from build123d import *

# Parameters (mm, degrees)
SKETCH1_R           = 45
BOSS_EXTRUDE1_DEPTH = 10
SKETCH3_R           = 2.1
CUT_EXTRUDE2_DEPTH  = 65.420493634
CIRPATTERN1_COUNT   = 4
SKETCH4_W           = 20
SKETCH4_H           = 20
CUT_EXTRUDE3_DEPTH  = 10
SKETCH6_R           = 2.55
CUT_EXTRUDE4_DEPTH  = 65.420493634


with BuildPart() as part:
    # Sketch1 → Boss-Extrude1 (new body)
    with BuildSketch(Plane(origin=(0, 0, 0), x_dir=(1, 0, 0), z_dir=(0, 1, 0))):
        with Locations(Location((0, 0, 0), (0, 0, 270))):
            Circle(SKETCH1_R)
    extrude(amount=BOSS_EXTRUDE1_DEPTH)

    # Sketch3 → Cut-Extrude2 (cut, through all)
    with BuildSketch(Plane(origin=(0, 10, 0), x_dir=(1, 0, 0), z_dir=(0, 1, 0))):
        with Locations(Location((0, 25, 0), (0, 0, 270))):
            Circle(SKETCH3_R)
    cut_extrude2 = extrude(amount=-CUT_EXTRUDE2_DEPTH, mode=Mode.SUBTRACT)

    # CirPattern1: Cut-Extrude2 ×4 about axis
    cirpattern1_axis = Axis((0, 0, 0), (0, 1, 0))
    for i in range(1, CIRPATTERN1_COUNT):
        add(cut_extrude2.rotate(cirpattern1_axis, i * 360 / CIRPATTERN1_COUNT), mode=Mode.SUBTRACT)

    # Sketch4 → Cut-Extrude3 (cut)
    with BuildSketch(Plane(origin=(0, 10, 0), x_dir=(1, 0, 0), z_dir=(0, 1, 0))):
        Rectangle(SKETCH4_W, SKETCH4_H)
    extrude(amount=-CUT_EXTRUDE3_DEPTH, mode=Mode.SUBTRACT)

    # Sketch6 → Cut-Extrude4 (cut, through all)
    with BuildSketch(Plane(origin=(0, 10, 0), x_dir=(1, 0, 0), z_dir=(0, 1, 0))):
        with Locations(Location((-26.516504294, 26.516504294, 0), (0, 0, 270))):
            Circle(SKETCH6_R)
        with Locations(Location((26.516504294, 26.516504294, 0), (0, 0, 270))):
            Circle(SKETCH6_R)
        with Locations(Location((26.516504294, -26.516504294, 0), (0, 0, 270))):
            Circle(SKETCH6_R)
        with Locations(Location((-26.516504294, -26.516504294, 0), (0, 0, 270))):
            Circle(SKETCH6_R)
    extrude(amount=-CUT_EXTRUDE4_DEPTH, mode=Mode.SUBTRACT)


solid = part.part
The listing builds one solid part. Answer for the finished solid, in the listing's coordinates (mm). A direction names the side the tool comes from. Coordinates: 2 decimals unless noted, no trailing zeros. Loops run counter-clockwise (first coordinate to the right, second up) from the corner with the lowest first, then second, coordinate; pieces in that order, holes last. Notation, with made-up numbers: (63, -2) -> (83, -2) arc R19 cw to (83, 5) -> close; hole circle Ø2 at (-35, 14). An arc over 180 degrees is marked (long way). Answer in a Markdown table with one row per item. Add a question column.
1. The part is cut by section B-B, the plane z = 0. Write down the section's boundary in (x, y).
2. The part is cut by section C-C, the plane y = 5. Count the separate pieces of the cut face and the enclosed holes in it, then the cut area to 3 significant figures.
3. Flat-ended cylindrical pins translate along their axes: P1, Ø4, axis at x = 26.52, z = 26.52, coming from the +Y side; P2, Ø4, axis at x = -33.5, y = 6, coming from the -Z side; P3, Ø4, axis at x = 17.5, y = 8, coming from the -Z side; P4, Ø6, axis at x = 27.5, y = 6, coming from the -Z side. Find the tip coordinate at first contact, or state that the pin passes through.
4. Determine the mould class of faces 3 (the flat face through (11, 0, -1)), 4 (the flat face through (10, 5, 0)), 5 (the cylindrical face through (-0.8, 5.07, -23.06)), 6 (the cylindrical face through (-17.235, 4.93, 41.569)) for opening direction Z: +Z half, -Z half, draft (parallel to the pull), parting line (faces both ways), or undercut.
5. Consider line 1 (X direction, y = 3.5, z = 25); line 2 (X direction, y = 4.25, z = -4). Determine where each line is inside the solid, lowest interval first. Write a range as [from, to].
6. The part is cut by section D-D, the plane z = -17. Write down the section's boundary in (x, y).
7. For faces 1 (the flat face through (0, 5, 10)), 2 (the flat face through (11, 10, -1)), determine the directions among +Z, -Z, +X, -X, +Y, -Y from which every point of the face is accessible in a straight line to the end or side of a thin tool.
8. The part is cut by section A-A, the plane x = 0. Write down the section's boundary in (y, z), then the cut area to 3 significant figures.
Answer below:
| question | item | result |
|---|---|---|
| 1 | outline | (-45, 0) -> (-27.1, 0) -> (-27.1, 10) -> (-45, 10) -> close; (-22.9, 0) -> (-10, 0) -> (-10, 10) -> (-22.9, 10) -> close; (10, 0) -> (22.9, 0) -> (22.9, 10) -> (10, 10) -> close; (27.1, 0) -> (45, 0) -> (45, 10) -> (27.1, 10) -> close |
| 2 | separate pieces | 1 |
| 2 | enclosed holes | 9 |
| 2 | area | 5,820 mm2 |
| 3 | P1 | through |
| 3 | P2 | z = -32.14 |
| 3 | P3 | z = -42.25 |
| 3 | P4 | z = -37.75 |
| 4 | face 3 | draft |
| 4 | face 4 | undercut |
| 4 | face 5 | undercut |
| 4 | face 6 | parting line |
| 5 | line 1 | [-37.42, -28.57], [-24.47, -2.1], [2.1, 24.47], [28.57, 37.42] |
| 5 | line 2 | [-44.82, -10], [10, 44.82] |
| 6 | outline | (-41.67, 0) -> (41.67, 0) -> (41.67, 10) -> (-41.67, 10) -> close |
| 7 | face 1 | +Y, -Y |
| 7 | face 2 | +Z, -Z, +X, -X, +Y |
| 8 | outline | (0, -45) -> (10, -45) -> (10, -27.1) -> (0, -27.1) -> close; (0, -22.9) -> (10, -22.9) -> (10, -10) -> (0, -10) -> close; (0, 10) -> (10, 10) -> (10, 22.9) -> (0, 22.9) -> close; (0, 27.1) -> (10, 27.1) -> (10, 45) -> (0, 45) -> close |
| 8 | area | 616 mm2 |
